Model file for the job. Use its own axes, mm. Face numbers are marked on the shaded views. A direction names the side the tool comes from. Round coordinates to 2 decimals unless told otherwise and drop trailing zeros. Order: outer loops, then holes, each group sorted by start corner. A loop starts at its lowest first (then second) coordinate and runs counter-clockwise, first axis right, second up. Notation, with made-up numbers: (-36.5, -19) - (-0.5, -19) arc R19 cw to (-0.5, -10) - close; hole circle Ø8 at (-8, 25.5). An arc over 180 degrees is marked (long way). Write item = value, one per line.
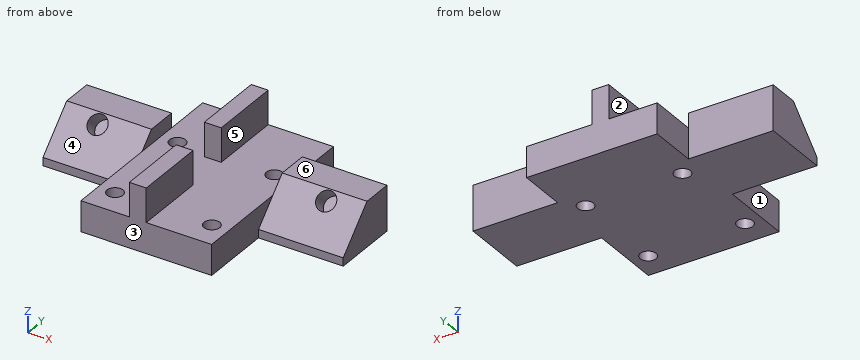
```python
from build123d import *

# Parameters (mm, degrees)
SKETCH_1_R             = 1.65
EXTRUDE_512_DEPTH      = 13.3
CUT_EXTRUDE_925_DEPTH  = 7
SKETCH_3_W             = 17.5
SKETCH_3_H             = 14
CUT_EXTRUDE_1164_DEPTH = 4
CUT_EXTRUDE_R_DEPTH    = 17.5
CUT_EXTRUDE_L_DEPTH    = 17.5
SKETCH_6_R             = 2
CUT_EXTRUDE_5_DEPTH    = 3.5


with BuildPart() as part:
    # Эскиз1 → Extrude 512 (new body)
    with BuildSketch(Plane.XY):
        Polygon((-13.5, 23.5), (13.5, 23.5), (13.5, 13.5), (31, 13.5), (31, -0.5), (13.5, -0.5), (13.5, -15.5), (-13.5, -15.5), (-13.5, -0.5), (-31, -0.5), (-31, 13.5), (-13.5, 13.5), align=None)
        with Locations((-10, 10)):
            Circle(SKETCH_1_R, mode=Mode.SUBTRACT)
        with Locations((10, 10)):
            Circle(SKETCH_1_R, mode=Mode.SUBTRACT)
        with Locations((10, -10)):
            Circle(SKETCH_1_R, mode=Mode.SUBTRACT)
        with Locations((-10, -10)):
            Circle(SKETCH_1_R, mode=Mode.SUBTRACT)
    extrude(amount=EXTRUDE_512_DEPTH)

    # Эскиз2 → Cut-Extrude 925 (cut)
    with BuildSketch(Plane.XY.offset(13.3)):
        Polygon((0, 23.5), (13.5, 23.5), (13.5, -15.5), (0, -15.5), (0, -0.5), (-3.5, -0.5), (-3.5, -15.5), (-13.5, -15.5), (-13.5, 23.5), (-3.5, 23.5), (-3.5, 8.5), (0, 8.5), align=None)
    extrude(amount=-CUT_EXTRUDE_925_DEPTH, mode=Mode.SUBTRACT)

    # Эскиз3 → Cut-Extrude 1164 (cut)
    with BuildSketch(Plane.XY.offset(13.3)):
        with Locations((-22.25, 6.5)):
            Rectangle(SKETCH_3_W, SKETCH_3_H)
        with Locations((22.25, 6.5)):
            Rectangle(SKETCH_3_W, SKETCH_3_H)
    extrude(amount=-CUT_EXTRUDE_1164_DEPTH, mode=Mode.SUBTRACT)

    # Эскиз4 → СрезТягиR (cut)
    with BuildSketch(Plane(origin=(31, 0, 0), x_dir=(0, 0, -1), z_dir=(1, 0, 0))):
        Polygon((-9.3, 7.1), (-1.7, -0.5), (-9.3, -0.5), align=None)
    extrude(amount=-CUT_EXTRUDE_R_DEPTH, mode=Mode.SUBTRACT)

    # Эскиз5 → СрезТягиL (cut)
    with BuildSketch(Plane.ZY.offset(31)):
        Polygon((9.3, 7.1), (9.3, -0.5), (1.7, -0.5), align=None)
    extrude(amount=-CUT_EXTRUDE_L_DEPTH, mode=Mode.SUBTRACT)

    # Эскиз6 → Вырез-Вытянуть5 (cut)
    with BuildSketch(Plane(origin=(0, -1.1, 1.1), x_dir=(1, 0, 0), z_dir=(0, -0.7071067811865472, 0.7071067811865478))):
        with Locations(Location((-23.605, 9.348528137, 0), (0, 0, 270))):
            Circle(SKETCH_6_R)
        with Locations(Location((23.605, 9.348528137, 0), (0, 0, 270))):
            Circle(SKETCH_6_R)
    extrude(amount=-CUT_EXTRUDE_5_DEPTH, mode=Mode.SUBTRACT)


solid = part.part
```
1) Cut at B-B (z = 2.5). Write the cut outline in (x, y), and give its area (3 significant figures).
Conclusion:
outline = (-31, 0.3) - (-13.5, 0.3) - (-13.5, -15.5) - (13.5, -15.5) - (13.5, 0.3) - (31, 0.3) - (31, 13.5) - (13.5, 13.5) - (13.5, 23.5) - (-13.5, 23.5) - (-13.5, 13.5) - (-31, 13.5) - close; hole circle Ø3.3 at (-10, -10); hole circle Ø3.3 at (-10, 10); hole circle Ø3.3 at (10, -10); hole circle Ø3.3 at (10, 10)
area = 1,480 mm^2
2) Cut at D-D (y = -10). Write the cut outline in (x, z), and give its area (3 significant figures).
Conclusion:
outline = (-13.5, 0) - (-11.65, 0) - (-11.65, 6.3) - (-13.5, 6.3) - close; (-8.35, 0) - (8.35, 0) - (8.35, 6.3) - (0, 6.3) - (0, 13.3) - (-3.5, 13.3) - (-3.5, 6.3) - (-8.35, 6.3) - close; (11.65, 0) - (13.5, 0) - (13.5, 6.3) - (11.65, 6.3) - close
area = 153 mm^2
3) Flat gauge pins, fed straight in: pin 1 Ø1.9 at (x, y) = (-26.5, 12) entering from +Z; pin 2 Ø3 at (y, z) = (16.5, 2.5) entering from +X; pin 3 Ø5 at (y, z) = (-6, 4) entering from -X. Where does each tip first touch, or does it go through?
Conclusion:
pin_1 = 9.3
pin_2 = 13.5
pin_3 = -13.5
4) Cut at A-A (z = 12). Write the cut outline in (x, y), and give its area (3 significant figures).
Conclusion:
outline = (-3.5, -15.5) - (0, -15.5) - (0, -0.5) - (-3.5, -0.5) - close; (-3.5, 8.5) - (0, 8.5) - (0, 23.5) - (-3.5, 23.5) - close
area = 105 mm^2
5) Mould opens along X. For the marked faces 1, 2 and 3 say: +X half, -X half, draft (parallel to the pull), parting line (faces both ways), or undercut.
Conclusion:
face_1 = -X half
face_2 = undercut
face_3 = draft
6) 3-axis set-ups, long thin cutter, end or side, ignore diameter. For the marked faces 4, 5 and 6: which of +Z, -Z, +X, -X, +Y, -Y reach the whole face in a straight line?
Conclusion:
face_4 = +Z, -X, -Y
face_5 = +Z, +Y, -Y
face_6 = +Z, +X, +Y, -Y
7) Cut at C-C (x = 10). Write the cut outline in (y, z).
Conclusion:
outline = (-15.5, 0) - (-11.65, 0) - (-11.65, 6.3) - (-15.5, 6.3) - close; (-8.35, 0) - (8.35, 0) - (8.35, 6.3) - (-8.35, 6.3) - close; (11.65, 0) - (23.5, 0) - (23.5, 6.3) - (11.65, 6.3) - close
8) Wall check: line 1 along Y through (x, z) = (10, 2.75); line 2 along X through (y, z) = (10, 5.25); line 3 along X through (y, z) = (-10, 3). Give the ranges that are in metal, low to high.
Conclusion:
line_1 = -15.5 to -11.65, -8.35 to 8.35, 11.65 to 23.5
line_2 = -31 to -11.65, -8.35 to 8.35, 11.65 to 31
line_3 = -13.5 to -11.65, -8.35 to 8.35, 11.65 to 13.5
